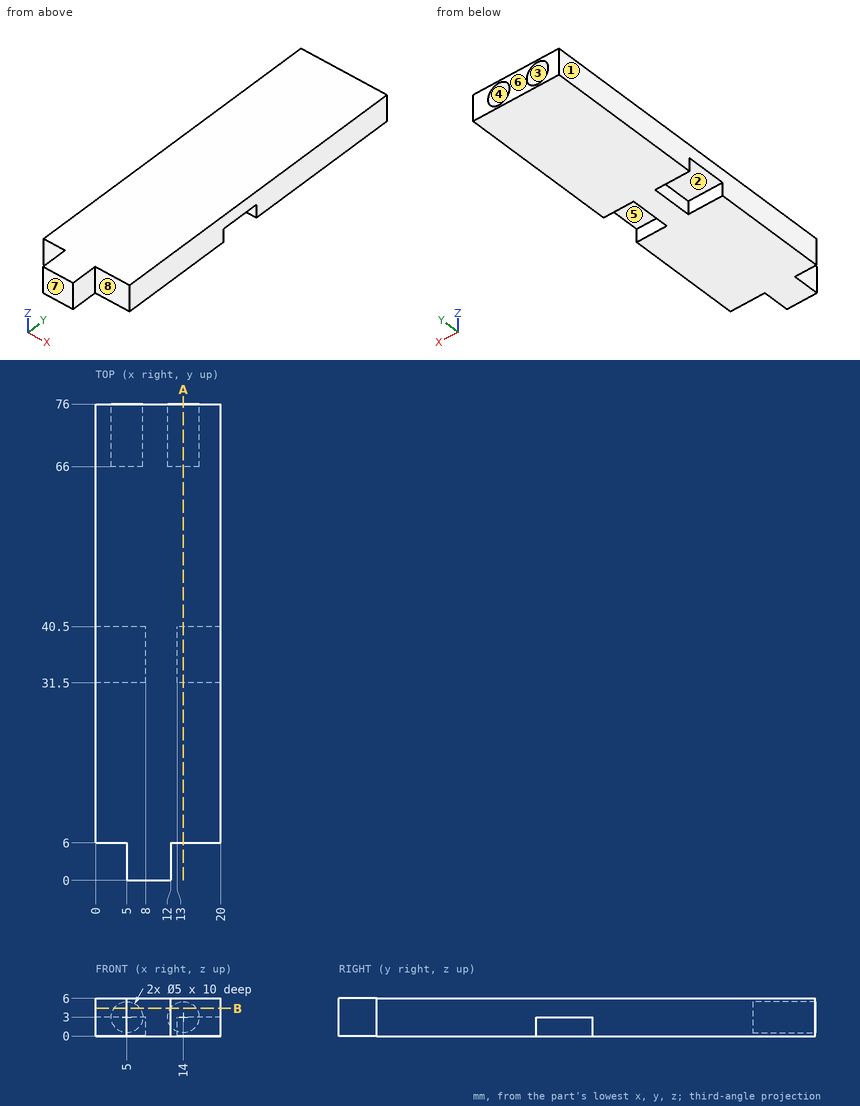
For this review, use the dimensioned drawing (mm, ordinates from the lowest corner) and the shaded views. A direction names the side the tool comes from. Round coordinates to 2 decimals unless told otherwise and drop trailing zeros. Write each loop counter-clockwise with the first axis right and the second up, starting at its lowest first coordinate (ties: lowest second). Pieces come first, ordered by that corner, then holes. Notation, with made-up numbers: (57.25, 20.25) -> (89.25, 20.25) arc R23 ccw to (89.25, 42.25) -> close; hole circle Ø9 at (20, 40.5). An arc over 180 degrees is marked (long way). Use CSV: the item, a comma, the result in double quotes.
(1) To check wall thickness, follow L1, parallel to X at y = 73.5, z = 3; L2, parallel to Y at x = 16, z = 2.35; L3, parallel to Y at x = 7.25, z = 2.2. State the ranges of each line that lie inside material, in increasing order. Write a range as [from, to].
Computed values:
L1,"[0, 2.5], [7.5, 11.5], [16.5, 20]"
L2,"[6, 31.5], [40.5, 66]"
L3,"[0, 31.5], [40.5, 66]"
(2) Consider section A-A, the plane x = 14. Give the boundary of the cut face in (y, z), plus the area to 3 significant figures.
Computed values:
outline,"(6, 0) -> (31.5, 0) -> (31.5, 3) -> (40.5, 3) -> (40.5, 0) -> (76, 0) -> (76, 0.5) -> (66, 0.5) -> (66, 5.5) -> (76, 5.5) -> (76, 6) -> (6, 6) -> close"
area,"343 mm²"
(3) Consider section B-B, the plane z = 4.4. Give the boundary of the cut face in (x, y), plus the area to 3 significant figures.
Computed values:
outline,"(0, 6) -> (5, 6) -> (5, 0) -> (12, 0) -> (12, 6) -> (20, 6) -> (20, 76) -> (16.07, 76) -> (16.07, 66) -> (11.93, 66) -> (11.93, 76) -> (7.07, 76) -> (7.07, 66) -> (2.93, 66) -> (2.93, 76) -> (0, 76) -> close"
area,"1,360 mm²"
(4) For the marked faces 4, 5, 6, 7 and 8, list the 3-axis set-ups (+Z, -Z, +X, -X, +Y, -Y) from which the entire face can be reached by the end or side of a thin tool; tool diameter is ignored.
Computed values:
face 4,"+Y"
face 5,"-Z, +X"
face 6,"+Z, -Z, +X, -X, +Y"
face 7,"+Z, -Z, +X, -X, -Y"
face 8,"+Z, -Z, +X, -Y"
(5) Clearance check with flat-ended pins moving along their axes: P1, Ø3, axis at x = 5, z = 3, coming from the +Y side; P2, Ø3.5, axis at x = 17, y = 37.5, coming from the -Z side; P3, Ø1.8, axis at y = 3.5, z = 3, coming from the -X side. State where each tip first meets the part, or that it passes through.
Computed values:
P1,"y = 66"
P2,"z = 3"
P3,"x = 5"
(6) Draft analysis for pull direction Z (two halves, no side actions). For the marked faces 1, 2 and 3, state which applies: +Z half, -Z half, draft (parallel to the pull), parting line (faces both ways), or undercut.
Computed values:
face 1,"draft"
face 2,"-Z half"
face 3,"undercut"
